```python
from build123d import *

# Parameters (mm, degrees)
CIRPATTERN1_COUNT = 12


with BuildPart() as part:
    # Sketch1 → Revolve1 (revolve)
    with BuildSketch(Plane.XY):
        Polygon((-76.2, 0), (-76.2, 25.4), (-50.8, 25.4), (-31.75, 31.75), (-12.7, 31.75), (-12.7, 25.4), (-31.75, 15.875), (-31.75, 12.7), (-33.3375, 12.7), (-33.3375, 14.732), (-36.0807, 14.732), (-36.0807, 12.7), (-50.8, 12.7), (-50.8, 0), (-52.3875, 0), (-52.3875, 2.032), (-55.1307, 2.032), (-55.1307, 0), align=None)
    revolve(axis=Axis((0, -1.5875, 0), (0, 1, 0)))

    # Sketch3 → 3/8 (0.375) Diameter Hole1 (revolve, cut)
    with BuildSketch(Plane(origin=(-63.5, 25.4, 0), x_dir=(0, 0, 1), z_dir=(1, 0, 0))):
        Polygon((0, 0), (0, 53.661598698), (4.7625, 50.8), (4.7625, 0), align=None)
    f_3_8_0_375_diameter_hole1 = revolve(axis=Axis((-63.5, 31.75, 0), (0, -1, 0)), mode=Mode.SUBTRACT)

    # CirPattern1: 3/8 (0.375) Diameter Hole1 ×12 about axis
    cirpattern1_axis = Axis((0, 0, 0), (0, 1, 0))
    for i in range(1, CIRPATTERN1_COUNT):
        add(f_3_8_0_375_diameter_hole1.rotate(cirpattern1_axis, i * 360 / CIRPATTERN1_COUNT), mode=Mode.SUBTRACT)


solid = part.part
```
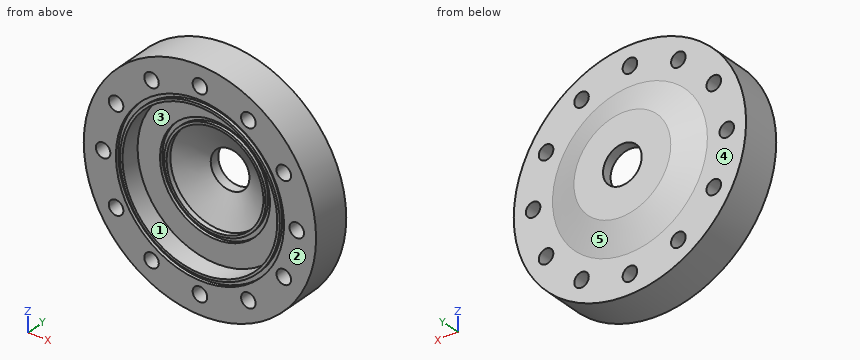
Design review of the part built by this model. Coordinates are the model's own, in mm. Face numbers are marked on the shaded views. A direction names the side the tool comes from. Coordinates: 2 decimals unless noted, no trailing zeros. Loops run counter-clockwise (first coordinate to the right, second up) from the corner with the lowest first, then second, coordinate; pieces in that order, holes last.
Q1. For pin 1 (8 mm diameter, centred on x = 37.5, y = 28, fed in from +Z); pin 2 (3 mm diameter, centred on y = 20, z = 43.5, fed in from -X); pin 3 (4 mm diameter, centred on x = -20, z = -55.5, fed in from +Y), all flat-tipped, find the tip position at first contact; note any pin that passes through.
Reported:
pin 1: stops at z = 67.96
pin 2: stops at x = -63.58
pin 3: stops at y = 25.4
Q2. We need section A-A on z = 63.5. State the section outline as (x, y) points, and give its area (3 significant figures).
Reported:
outline: (-42.12, 0) - (-4.76, 0) - (-4.76, 25.4) - (-42.12, 25.4) - close; (4.76, 0) - (42.12, 0) - (42.12, 25.4) - (4.76, 25.4) - close
area: 1,900 mm2
Q3. We need section C-C on y = 20.5. State how many separate pieces and enclosed holes the cut face has, and give its area (3 significant figures).
Reported:
separate pieces: 1
enclosed holes: 13
area: 15,800 mm2
Q4. We need section B-B on x = -63.5. State the section outline as (y, z) points.
Reported:
outline: (0, -42.12) - (25.4, -42.12) - (25.4, -4.76) - (0, -4.76) - close; (0, 4.76) - (25.4, 4.76) - (25.4, 42.12) - (0, 42.12) - close
Q5. The part is to be moulded in two halves that separate along X. For the marked faces 3, 4 and 5, say which applies: +X half, -X half, draft (parallel to the pull), parting line (faces both ways), or undercut.
Reported:
face 3: undercut
face 4: draft
face 5: parting line
Q6. Tool access review of the marked faces 1 and 2: name each direction out of +Z, -Z, +X, -X, +Y, -Y from which nothing blocks a thin tool from reaching the whole face with its end or side.
Reported:
face 1: -Y
face 2: +Z, -Z, +X, -X, -Y
Q7. To check wall thickness, follow line 1 (Z direction, x = 0.5, y = 12.5); line 2 (Z direction, x = 0, y = 14.95); line 3 (Z direction, x = -58, y = 3.5). State the ranges of each line that lie inside material, in increasing order.
Reported:
line 1: z = -76.2 to -68.24, -58.76 to -50.8, 50.8 to 58.76, 68.24 to 76.2
line 2: z = -76.2 to -68.26, -58.74 to -31.75, 31.75 to 58.74, 68.26 to 76.2
line 3: z = -49.42 to -35.44, -28.06 to 28.06, 35.44 to 49.42
